The listing builds one solid part. Answer for the finished solid, in the listing's coordinates (mm). A direction names the side the tool comes from. Round coordinates to 2 decimals unless told otherwise and drop trailing zeros. Loops run counter-clockwise (first coordinate to the right, second up) from the corner with the lowest first, then second, coordinate; pieces in that order, holes last. Notation, with made-up numbers: M -29.75,-34 L -24.75,-34 A19 ccw -24.75,-24 Z; hole C -30,29 d11. An arc over 180 degrees is marked long. Answer as a JSON object with one key per item and string values.
```python
from build123d import *

# Parameters (mm, degrees)
EXTRUDE_1_DEPTH     = 74
SKETCH_2_W          = 9.512991355
SKETCH_2_H          = 18
CUT_EXTRUDE_1_DEPTH = 102.843016452


with BuildPart() as part:
    # Эскиз1 → Вытянуть1 (new body)
    with BuildSketch(Plane(origin=(0, 0, 0), x_dir=(0, 0, -1), z_dir=(1, 0, 0))):
        Polygon((0, 0), (0, 60), (-4, 60), (-4, -5), (36, -5), (36, 0), align=None)
    extrude(amount=-EXTRUDE_1_DEPTH)

    # Эскиз2 → Вырез-Вытянуть1 (cut, through all)
    with BuildSketch(Plane(origin=(0, 0, 0), x_dir=(1, 0, 0), z_dir=(0, 1, 0))):
        Polygon((-33.857381994, 16), (-69.85538749, 16), (-69.85538749, 0), (-75.857381994, 0), (-75.857381994, 39.592922538), (-33.857381994, 39.592922538), align=None)
        with Locations((-4.756495678, 27)):
            Rectangle(SKETCH_2_W, SKETCH_2_H)
    extrude(amount=-CUT_EXTRUDE_1_DEPTH, mode=Mode.SUBTRACT)


solid = part.part
```
Item 1: The part is cut by section B-B (z = -33). Give the vertices of the cut face in (x, y).
Values follow:
{"outline": "M -33.86,-5 L -9.51,-5 L -9.51,0 L -33.86,0 Z"}
Item 2: The part is cut by section A-A (x = -15). Give the vertices of the cut face in (y, z).
Values follow:
{"outline": "M -5,-36 L 0,-36 L 0,0 L 60,0 L 60,4 L -5,4 Z"}
Item 3: The part is cut by section C-C (y = 27). Give the vertices of the cut face in (x, z), then the cut area to 3 significant figures.
Values follow:
{"outline": "M -74,0 L 0,0 L 0,4 L -74,4 Z", "area": "296 mm^2"}
Item 4: Straight lines are drawn through the part: line 1 (Z direction, x = -27.5, y = 1.5); line 2 (Y direction, x = -22.5, z = -3.5); line 3 (X direction, y = -1, z = -1). For each, find the intervals that lie inside material, in ascending order.
Values follow:
{"line 1": "0 to 4", "line 2": "-5 to 0", "line 3": "-69.86 to 0"}
Item 5: The part is cut by section D-D (x = -58). Give the vertices of the cut face in (y, z), then the cut area to 3 significant figures.
Values follow:
{"outline": "M -5,-16 L 0,-16 L 0,0 L 60,0 L 60,4 L -5,4 Z", "area": "340 mm^2"}
Item 6: Flat-ended cylindrical pins translate along their axes: P1, Ø1.5, axis at x = -46.5, y = 23.5, coming from the -Z side; P2, Ø4, axis at y = -2, z = -29, coming from the +X side; P3, Ø5, axis at x = -30, z = -4, coming from the +Y side. Find the tip coordinate at first contact, or state that the pin passes through.
Values follow:
{"P1": "z = 0", "P2": "x = -9.51", "P3": "y = 0"}
Item 7: Which of the six approach directions +Z, -Z, +X, -X, +Y, -Y give full straight-line access (tool end or side, diameter ignored) to faces 1 (the face through (-36, -5, -11)), 2 (the face through (-36, 28, 4)), 3 (the face through (-69.855, -2, -8)), 4 (the face through (-27, 0, -14)), 5 (the face through (-9.513, -2, -27))?
Values follow:
{"face 1": "+Z, -Z, +X, -X, -Y", "face 2": "+Z, +X, -X, +Y, -Y", "face 3": "-Z, -X, +Y, -Y", "face 4": "-Z, +X, -X, +Y", "face 5": "-Z, +X, +Y, -Y"}
